```python
from build123d import *

# Parameters (mm, degrees)
SKETCH1_W                    = 81.28
SKETCH1_H                    = 101.6
BASE_FLANGE1_DEPTH           = 1.2192
EDGE_FLANGE1_STRIP_W         = 7.4168
EDGE_FLANGE1_STRIP_H         = 1.2192
EDGE_FLANGE1_STRIP_CUT_DEPTH = 101.6
EDGE_FLANGE1_DEPTH           = 101.6
EDGE_FLANGE2_STRIP_W         = 7.4168
EDGE_FLANGE2_STRIP_H         = 1.2192
EDGE_FLANGE2_STRIP_CUT_DEPTH = 101.6
EDGE_FLANGE2_DEPTH           = 101.6


# Sheet-metal steps are written as plain solids
with BuildPart() as part:
    # Sketch1 → Base-Flange1 (new body)
    with BuildSketch(Plane(origin=(0, 0, 0), x_dir=(0, 0, -1), z_dir=(1, 0, 0))):
        with Locations((40.64, 50.8)):
            Rectangle(SKETCH1_W, SKETCH1_H)
    extrude(amount=-BASE_FLANGE1_DEPTH)

    # Edge-Flange1 strip (across the edge) → Edge-Flange1 strip cut (cut)
    with BuildSketch(Plane(origin=(-1.2192, 0, 0), x_dir=(0, 0, -1), z_dir=(0, 1, 0))):
        with Locations((-1.2192, -0.6096)):
            Rectangle(EDGE_FLANGE1_STRIP_W, EDGE_FLANGE1_STRIP_H)
    extrude(amount=EDGE_FLANGE1_STRIP_CUT_DEPTH, mode=Mode.SUBTRACT)

    # Edge-Flange1 section (across the edge) → Edge-Flange1 (add)
    with BuildSketch(Plane(origin=(-1.2192, 0, 0), x_dir=(0, 0, -1), z_dir=(0, 1, 0))):
        with BuildLine():
            Line((0, 1.27), (0, 74.9808))
            Line((0, 74.9808), (1.2192, 74.9808))
            Line((1.2192, 74.9808), (1.2192, 1.27))
            ThreePointArc((1.2192, 1.27), (1.591174388, 0.371974388), (2.4892, 0))
            Line((2.4892, 0), (2.4892, -1.2192))
            ThreePointArc((2.4892, -1.2192), (0.7290698, -0.4901302), (0, 1.27))
        make_face()
    extrude(amount=EDGE_FLANGE1_DEPTH)

    # Edge-Flange2 strip (across the edge) → Edge-Flange2 strip cut (cut)
    with BuildSketch(Plane(origin=(-1.2192, 101.6, -81.28), x_dir=(0, 0, 1), z_dir=(0, -1, 0))):
        with Locations((-1.2192, -0.6096)):
            Rectangle(EDGE_FLANGE2_STRIP_W, EDGE_FLANGE2_STRIP_H)
    extrude(amount=EDGE_FLANGE2_STRIP_CUT_DEPTH, mode=Mode.SUBTRACT)

    # Edge-Flange2 section (across the edge) → Edge-Flange2 (add)
    with BuildSketch(Plane(origin=(-1.2192, 101.6, -81.28), x_dir=(0, 0, 1), z_dir=(0, -1, 0))):
        with BuildLine():
            Line((0, 1.27), (0, 74.9808))
            Line((0, 74.9808), (1.2192, 74.9808))
            Line((1.2192, 74.9808), (1.2192, 1.27))
            ThreePointArc((1.2192, 1.27), (1.591174388, 0.371974388), (2.4892, 0))
            Line((2.4892, 0), (2.4892, -1.2192))
            ThreePointArc((2.4892, -1.2192), (0.7290698, -0.4901302), (0, 1.27))
        make_face()
    extrude(amount=EDGE_FLANGE2_DEPTH)


solid = part.part
```
Geometry: final body of the model. Coordinates: model frame, mm. A direction names the side the tool comes from. Give positions to 0.01 mm unless a question says otherwise; leave off trailing zeros. Order: outer loops, then holes, each group sorted by start corner. A loop starts at its lowest first (then second) coordinate and runs counter-clockwise, first axis right, second up. Notation, with made-up numbers: M -36.75,-6 L -32.75,-6 A28 cw -32.75,19 Z; hole C 5.25,46.25 d10. An arc over 180 degrees is marked long. Answer as CSV lines item,"result". Start each with the question number.
1) Mould query, pull axis Z, two halves, no side actions, for faces 3 (the flat face through (-1.219, 52, -40)), 4 (the flat face through (-40, 50, -1.219)), 5 (the flat face through (-39, 52, -81.28)), 6 (the cylindrical face through (-0.71, 50.09, -0.75)). Classes: +Z half, -Z half, draft (parallel to the pull), parting line (faces both ways), or undercut.
2) Set-up query: faces 1 (the flat face through (-40, 52, -80.061)), 2 (the flat face through (-39, 50, 0)). Return all of +Z, -Z, +X, -X, +Y, -Y with unobstructed straight access to the full face (end or side cutting, diameter ignored); none if empty.
3) Cut plane B-B (y = 36). Output: boundary loops of the cut face in (x, z), then the cut area to 3 significant figures.
4) Line query: line 1 (Z direction, x = -68, y = 96); line 2 (X direction, y = 68.5, z = -20). Output: solid intervals per line, ascending. Write a range as from..to.
5) Cut plane C-C (z = -19). Output: boundary loops of the cut face in (x, y).
6) First-contact query: P1, Ø3, axis at y = 49.5, z = -23, coming from the +X side. Flat tip, straight axial feed; report the tip coordinate or a pass-through.
7) Cut plane A-A (x = -49). Output: boundary loops of the cut face in (y, z).
Findings below:
1,face 3,"undercut"
1,face 4,"undercut"
1,face 5,"-Z half"
1,face 6,"+Z half"
2,face 1,"-X, +Y, -Y"
2,face 2,"+Z, +X, -X, +Y, -Y"
3,outline,"M -76.2,-81.28 L -2.49,-81.28 A2.49 ccw 0,-78.79 L 0,-2.49 A2.49 ccw -2.49,0 L -76.2,0 L -76.2,-1.22 L -2.49,-1.22 A1.27 cw -1.22,-2.49 L -1.22,-78.79 A1.27 cw -2.49,-80.06 L -76.2,-80.06 Z"
3,area,"280 mm²"
4,line 1,"z = -81.28..-80.06, -1.22..0"
4,line 2,"x = -1.22..0"
5,outline,"M -1.22,0 L 0,0 L 0,101.6 L -1.22,101.6 Z"
6,P1,"stops at x = 0"
7,outline,"M 0,-81.28 L 101.6,-81.28 L 101.6,-80.06 L 0,-80.06 Z; M 0,-1.22 L 101.6,-1.22 L 101.6,0 L 0,0 Z"
